Read the model definition and answer for the solid it produces. Units are mm, in the model's axes. A direction names the side the tool comes from. Give positions to 0.01 mm unless a question says otherwise; leave off trailing zeros. Loops run counter-clockwise (first coordinate to the right, second up) from the corner with the lowest first, then second, coordinate; pieces in that order, holes last.
(1) Find section A-A, the plane z = 2.5. Write down the section's boundary in (x, y).
(2) Each of these flat-tipped pins is pushed along its axis until it touches: P1, Ø4, axis at y = 3, z = -7, coming from the +X side; P2, Ø2, axis at x = -20, y = 2.5, coming from the -Z side; P3, Ø5, axis at x = -6.5, z = -12, coming from the +Y side; P4, Ø0.6, axis at y = 2, z = 2.5, coming from the -X side. Where does it stop, or does it pass through?
(3) Find section C-C, the plane y = -3.5. Write down the section's boundary in (x, z), then the cut area to 3 significant figures.
(4) Which of the six approach directions +Z, -Z, +X, -X, +Y, -Y give full straight-line access (tool end or side, diameter ignored) to faces 1 (the face through (14.14, 0.9, 0.74)), 2 (the face through (-25, 4, 2)), 3 (the face through (-22.75, 4, 2)), 4 (the face through (21, 4, 5))?
(5) Find section B-B, the plane x = 19. State how many separate pieces and enclosed holes the cut face has, then the cut area to 3 significant figures.
(6) Determine the mould class of faces 5 (the face through (25.865, -3.479, 13.224)), 6 (the face through (-17, 3, 3.5)), 7 (the face through (-21, 4, 5)) for opening direction X: pulls with the +X half, pulls with the -X half, needs draft (parallel to the pull), parting line crosses it, or undercut.
(7) Straight lines are drawn through the part: probe 1 along Y at (x, z) = (19, 4); probe 2 along X at (y, z) = (3.5, 4.55); probe 3 along Z at (x, y) = (-21, 6). For each, find the intervals that lie inside material, in ascending order.
Autodesk Inventor part; units mm, degrees
ref_plane "YZ Plane" through (0, 0, 0) normal (1, 0, 0) x (0, 1, 0)
ref_plane "XZ Plane" through (0, 0, 0) normal (0, 1, 0) x (-1, 0, 0)
ref_plane "XY Plane" through (0, 0, 0) normal (0, 0, 1) x (1, 0, 0)
sketch "Sketch1" plane through (0, 0, 0) normal (0, 0, 1) x (1, 0, 0)
  line L0 (25, 7) -> (-25, 7)
  line L1 (-25, 7) -> (-25, 0)
  line L2 (-25, 0) -> (25, 0)
  line L3 (25, 0) -> (25, 7)
  circle A0 centre (-19, 3.5) radius 1.6
  circle A1 centre (19, 3.5) radius 1.6
  line L4 (19, 3.5) -> (-19, 3.5) construction
  line L5 (19, 3.5) -> (25, 7) construction
  line L6 (19, 3.5) -> (25, 0) construction
  line L7 (-19, 3.5) -> (-25, 7) construction
  line L8 (-19, 3.5) -> (-25, 0) construction
  line L9 (0, 0) -> (-19, 3.5) construction
  line L10 (0, 0) -> (19, 3.5) construction
  dimension "d0" = 3.2
  dimension "d1" = 38
  dimension "d2" = 7
  dimension "d3" = 50
extrude "Extrusion1" add sketch "Sketch1" along normal blind 5
sketch "Sketch2" plane through (-25, 7, 0) normal (0, 1, 0) x (1, 0, 0)
  line L0 (2.25, -3.5) -> (10, -3.5)
  line L1 (47.75, -3.5) -> (47.75, -1.5)
  line L2 (47.75, -1.5) -> (40, -1.5)
  line L3 (2.25, -1.5) -> (2.25, -3.5)
  line L4 (50, -5) -> (0, -5) construction
  line L5 (0, -5) -> (2.25, -3.5) construction
  line L6 (50, 0) -> (0, 0) construction
  line L7 (2.25, -1.5) -> (0, 0) construction
  line L8 (50, 0) -> (50, -5) construction
  line L9 (47.75, -3.5) -> (50, -5) construction
  line L10 (40, -3.5) -> (40, -5)
  line L11 (40, -5) -> (10, -5)
  line L12 (10, -5) -> (10, -3.5)
  line L13 (10, -1.5) -> (10, 0)
  line L14 (10, 0) -> (40, 0)
  line L15 (40, 0) -> (40, -1.5)
  line L16 (40, -3.5) -> (47.75, -3.5)
  line L17 (40, -1.5) -> (10, -1.5) construction
  line L18 (10, -3.5) -> (40, -3.5) construction
  line L19 (10, -1.5) -> (2.25, -1.5)
  line L20 (47.75, -3.5) -> (40, -5) construction
  line L21 (40, 0) -> (47.75, -1.5) construction
  line L22 (10, -5) -> (2.25, -3.5) construction
  line L23 (2.25, -1.5) -> (10, 0) construction
  point P0 (25, 0)
  dimension "d6" = 45.5
  dimension "d7" = 2
  dimension "d13" = 30
extrude "Extrusion2" cut sketch "Sketch2" against normal up to next
sketch "Sketch3" plane through (-25, 0, 0) normal (0, -1, 0) x (1, 0, 0)
  circle A0 centre (25, 2.5) radius 28
  line L0 (0, 5) -> (50, 5) construction
  line L1 (0, 5) -> (25, 2.5) construction
  line L2 (0, 0) -> (50, 0) construction
  line L3 (25, 2.5) -> (0, 0) construction
  line L4 (25, 2.5) -> (50, 5) construction
  point P0 (25, 0)
  dimension "d10" = 56
extrude "Extrusion3" add sketch "Sketch3" along normal blind 5
fillet "Fillet1" radius 3 8 edges at (15, 7, 0.75) (15, 7, 4.25) (15, 0, 4.25) (15, 0, 0.75) (-15, 0, 0.75) (-15, 7, 0.75) (-15, 7, 4.25) (-15, 0, 4.25)
fillet "Fillet2" radius 2 1 edges at (-28, 0, 2.5)
properties part number "Main PCB Base"
Entries:
1. outline: (-28, -5) - (28, -5) - (28, -2) arc R2 ccw to (26, 0) - (25, 0) - (25, 7) - (22.75, 7) - (22.75, 0) - (-22.75, 0) - (-22.75, 7) - (-25, 7) - (-25, 0) - (-26, 0) arc R2 ccw to (-28, -2) - close
2. P1: passes through
2. P2: stops at z = 0
2. P3: stops at y = 0
2. P4: stops at x = -25
3. outline: circle Ø56 at (0, 2.5)
3. area: 2,460 mm2
4. face 1: +Z, -Z, +Y
4. face 2: +Z, -Z, -X, +Y
4. face 3: +Y
4. face 4: +Z, +X, -X, +Y
5. separate pieces: 3
5. enclosed holes: 0
5. area: 215 mm2
6. face 5: parting line crosses it
6. face 6: undercut
6. face 7: needs draft
7. probe 1: y = -5 to 1.9, 5.1 to 7
7. probe 2: x = -25 to -20.6, -17.4 to -15, 15 to 17.4, 20.6 to 25
7. probe 3: z = 0 to 1.5, 3.5 to 5
